The listing builds one solid part. Answer for the finished solid, in the listing's coordinates (mm). A direction names the side the tool comes from. Round coordinates to 2 decimals unless told otherwise and drop trailing zeros. Order: outer loops, then holes, each group sorted by start corner. A loop starts at its lowest first (then second) coordinate and runs counter-clockwise, first axis right, second up. Notation, with made-up numbers: (-12, 43) - (29, 43) arc R8 ccw to (29, 57) - close; hole circle Ø4 at (74, 41.25). An arc over 180 degrees is marked (long way). Write item = value, one per line.
from build123d import *

# Parameters (mm, degrees)
F0_W      = 25.4
F0_H      = 19.05
F1_DEPTH  = 0.79375
F2_R      = 4.7625
F3_W      = 19.05
F3_H      = 15.875
F4_DEPTH  = 4.9276
F6_DEPTH  = 0.79375
F7_R      = 1.5875
F9_W      = 15.875
F9_H      = 14.2875
F10_DEPTH = 0.79375
F11_R     = 0.79374
F12_R     = 0.79375
F14_DEPTH = 25.4
F15_W     = 25.4
F15_H     = 4.7625
F16_DEPTH = 25.4


# Not quite as in the source:
# - two fillets or chamfers of one size are made in one step
# - a fillet or chamfer is up to 0.001 mm smaller than in the source, because OpenCascade refuses the exact size


with BuildPart() as f1:
    # F0 (on Front) → F1 (new body)
    with BuildSketch(Plane.XZ):
        Rectangle(F0_W, F0_H)
    extrude(amount=F1_DEPTH)

    # F2
    f2_edges = [f1.edges().sort_by_distance(p)[0] for p in [
        (12.7, -0.396875, -9.525),
        (-12.7, -0.396875, -9.525),
    ]]
    fillet(f2_edges, radius=F2_R)

    # F3 (on face) → F4 (cut)
    with BuildSketch(Plane.XZ.offset(0.79375)):
        with Locations((0, 1.5875)):
            Rectangle(F3_W, F3_H)
    extrude(amount=-F4_DEPTH, mode=Mode.SUBTRACT)

    # F5 (on face) → F6 (join)
    with BuildSketch(Plane.XZ.offset(0.79375)):
        Polygon((-15.875, 15.875), (-15.875, 9.525), (-12.7, 9.525), (-9.525, 9.525), (9.525, 9.525), (12.7, 9.525), (15.875, 9.525), (15.875, 15.875), align=None)
    extrude(amount=-F6_DEPTH)

    # F7
    f7_edges = [f1.edges().sort_by_distance(p)[0] for p in [
        (-15.875, -0.396875, 15.875),
        (15.875, -0.396875, 15.875),
        (15.875, -0.396875, 9.525),
        (-15.875, -0.396875, 9.525),
        (-9.525, -0.396875, -6.35),
        (9.525, -0.396875, -6.35),
    ]]
    fillet(f7_edges, radius=F7_R)

    # F9 (on face) → F10 (join)
    with BuildSketch(Plane.XZ.offset(0.79375)):
        with BuildLine():
            ThreePointArc((-14.2875, 15.875), (-15.4100320151, 15.4100320151), (-15.875, 14.2875))
            Line((-15.875, 14.2875), (-15.875, 11.1125))
            ThreePointArc((-15.875, 11.1125), (-15.4100320151, 9.9899679849), (-14.2875, 9.525))
            Line((-14.2875, 9.525), (-12.7, 9.525))
            Line((-12.7, 9.525), (-12.7, -4.7625))
            ThreePointArc((-12.7, -4.7625), (-11.3050960454, -8.1300960454), (-7.9375, -9.525))
            Line((-7.9375, -9.525), (7.9375, -9.525))
            ThreePointArc((7.9375, -9.525), (11.3050960454, -8.1300960454), (12.7, -4.7625))
            Line((12.7, -4.7625), (12.7, 9.525))
            Line((12.7, 9.525), (14.2875, 9.525))
            ThreePointArc((14.2875, 9.525), (15.4100320151, 9.9899679849), (15.875, 11.1125))
            Line((15.875, 11.1125), (15.875, 14.2875))
            ThreePointArc((15.875, 14.2875), (15.4100320151, 15.4100320151), (14.2875, 15.875))
            Line((14.2875, 15.875), (-14.2875, 15.875))
        make_face()
        with BuildLine():
            Line((-9.525, 9.525), (-7.9375, 9.525))
            Line((-7.9375, 9.525), (7.9375, 9.525))
            Line((7.9375, 9.525), (9.525, 9.525))
            Line((9.525, 9.525), (9.525, -4.7625))
            ThreePointArc((9.525, -4.7625), (9.0600320151, -5.8850320151), (7.9375, -6.35))
            Line((7.9375, -6.35), (-7.9375, -6.35))
            ThreePointArc((-7.9375, -6.35), (-9.0600320151, -5.8850320151), (-9.525, -4.7625))
            Line((-9.525, -4.7625), (-9.525, 9.525))
        make_face(mode=Mode.SUBTRACT)
        with Locations((0, 2.38125)):
            Rectangle(F9_W, F9_H)
    extrude(amount=-F10_DEPTH)

    # F11 (radius 0.79375 in the source; OpenCascade refuses exactly that, so slightly less here)
    f11_edges = [f1.edges().sort_by_distance(p)[0] for p in [
        (-7.9375, -0.396875, 9.525),
        (-9.525, -0.396875, 9.525),
        (7.9375, -0.396875, 9.525),
        (9.525, -0.396875, 9.525),
    ]]
    fillet(f11_edges, radius=F11_R)

    # F12
    f12_edges = [f1.edges().sort_by_distance(p)[0] for p in [
        (-7.9375, -0.396875, -4.7625),
        (7.9375, -0.396875, -4.7625),
    ]]
    fillet(f12_edges, radius=F12_R)

    # F13 (on face) → F14 (cut)
    with BuildSketch(Plane.XZ.offset(0.79375)):
        with BuildLine():
            Line((-17.2636155039, 7.9375), (-12.7, 7.9375))
            Line((-12.7, 7.9375), (-12.7, 9.525))
            Line((-12.7, 9.525), (-14.2875, 9.525))
            ThreePointArc((-14.2875, 9.525), (-15.4100320151, 9.9899679849), (-15.875, 11.1125))
            Line((-15.875, 11.1125), (-15.875, 14.2875))
            ThreePointArc((-15.875, 14.2875), (-15.4100320151, 15.4100320151), (-14.2875, 15.875))
            Line((-14.2875, 15.875), (-12.7, 15.875))
            Line((-12.7, 15.875), (-12.7, 16.6596230119))
            Line((-12.7, 16.6596230119), (-17.2636155039, 16.6596230119))
            Line((-17.2636155039, 16.6596230119), (-17.2636155039, 7.9375))
        make_face()
        with BuildLine():
            Line((-14.2875, 9.525), (-12.7, 9.525))
            Line((-12.7, 9.525), (-12.7, 15.875))
            Line((-12.7, 15.875), (-14.2875, 15.875))
            ThreePointArc((-14.2875, 15.875), (-15.4100320151, 15.4100320151), (-15.875, 14.2875))
            Line((-15.875, 14.2875), (-15.875, 11.1125))
            ThreePointArc((-15.875, 11.1125), (-15.4100320151, 9.9899679849), (-14.2875, 9.525))
        make_face()
        with BuildLine():
            Line((14.2875, 15.875), (12.7, 15.875))
            Line((12.7, 15.875), (12.7, 9.525))
            Line((12.7, 9.525), (14.2875, 9.525))
            ThreePointArc((14.2875, 9.525), (15.4100320151, 9.9899679849), (15.875, 11.1125))
            Line((15.875, 11.1125), (15.875, 14.2875))
            ThreePointArc((15.875, 14.2875), (15.4100320151, 15.4100320151), (14.2875, 15.875))
        make_face()
        with BuildLine():
            Line((12.7, 16.9361550361), (12.7, 15.875))
            Line((12.7, 15.875), (14.2875, 15.875))
            ThreePointArc((14.2875, 15.875), (15.4100320151, 15.4100320151), (15.875, 14.2875))
            Line((15.875, 14.2875), (15.875, 11.1125))
            ThreePointArc((15.875, 11.1125), (15.4100320151, 9.9899679849), (14.2875, 9.525))
            Line((14.2875, 9.525), (12.7, 9.525))
            Line((12.7, 9.525), (12.7, 7.9375))
            Line((12.7, 7.9375), (16.7191289365, 7.9375))
            Line((16.7191289365, 7.9375), (16.7191289365, 16.9361550361))
            Line((16.7191289365, 16.9361550361), (12.7, 16.9361550361))
        make_face()
    extrude(amount=-F14_DEPTH, mode=Mode.SUBTRACT)

    # F15 (on face) → F16 (cut)
    with BuildSketch(Plane.XZ.offset(0.79375)):
        with Locations((0, 13.49375)):
            Rectangle(F15_W, F15_H)
    extrude(amount=-F16_DEPTH, mode=Mode.SUBTRACT)


solid = f1.part
Q1. For faces 5 (the face through (9.048, -0.391, -5.897)), 6 (the face through (0, -0.794, 1)), determine the directions among +Z, -Z, +X, -X, +Y, -Y from which every point of the face is accessible in a straight line to the end or side of a thin tool.
Model answer:
face_5 = +Y, -Y
face_6 = +Z, -Z, +X, -X, -Y
Q2. Section B-B on z = 3.5 is taken. Determine the outline of the cut face in (x, y) (1 decimal).
Model answer:
outline = (-12.7, -0.8) - (-9.5, -0.8) - (-9.5, 0) - (-12.7, 0) - close; (-7.9, -0.8) - (7.9, -0.8) - (7.9, 0) - (-7.9, 0) - close; (9.5, -0.8) - (12.7, -0.8) - (12.7, 0) - (9.5, 0) - close
Q3. Determine the mould class of faces 1 (the face through (11.268, -0.402, -8.167)), 2 (the face through (0, 0, 1)), 3 (the face through (-11.342, -0.402, -8.093)), 4 (the face through (-9.072, -0.391, -5.873)) for opening direction X: released by +X, released by -X, zero draft, split by the parting line, or undercut.
Model answer:
face_1 = released by +X
face_2 = zero draft
face_3 = released by -X
face_4 = undercut
Q4. Find the intervals of material crossed by line 1 (X direction, y = -0.45, z = 0.5) (1 decimal); line 2 (Z direction, x = -11, y = -0.65); line 3 (Z direction, x = -10.25, y = -0.3), in increasing order. Write a range as from..to.
Model answer:
line_1 = -12.7..-9.5, -7.9..7.9, 9.5..12.7
line_2 = -8.41..11.11
line_3 = -8.93..11.11
